from build123d import *

# Parameters (mm, degrees)
SKETCH2_W           = 70
SKETCH2_H           = 50
BOSS_EXTRUDE1_DEPTH = 10
SKETCH3_R           = 4
CUT_EXTRUDE1_DEPTH  = 11
SKETCH4_R           = 2
CUT_EXTRUDE2_DEPTH  = 10
SKETCH5_R           = 8.5
CUT_EXTRUDE3_DEPTH  = 11.0000001


with BuildPart() as part:
    # Sketch2 → Boss-Extrude1 (new body)
    with BuildSketch(Plane(origin=(0, 0, 0), x_dir=(1, 0, 0), z_dir=(0, 1, 0))):
        Rectangle(SKETCH2_W, SKETCH2_H)
    extrude(amount=BOSS_EXTRUDE1_DEPTH)

    # Sketch3 → Cut-Extrude1 (cut, through all)
    with BuildSketch(Plane.XZ):
        with Locations((-25, 15)):
            Circle(SKETCH3_R)
        with Locations((25, 15)):
            Circle(SKETCH3_R)
    extrude(amount=-CUT_EXTRUDE1_DEPTH, mode=Mode.SUBTRACT)

    # Sketch4 → Cut-Extrude2 (cut)
    with BuildSketch(Plane.XY.offset(25)):
        with Locations((25, 5)):
            Circle(SKETCH4_R)
        with Locations((-25, 5)):
            Circle(SKETCH4_R)
    extrude(amount=-CUT_EXTRUDE2_DEPTH, mode=Mode.SUBTRACT)

    # Sketch5 → Cut-Extrude3 (cut, through all)
    with BuildSketch(Plane.XZ):
        with Locations((0, 4)):
            Circle(SKETCH5_R)
    extrude(amount=-CUT_EXTRUDE3_DEPTH, mode=Mode.SUBTRACT)


solid = part.part
Could you check a few things on this model? Use its own coordinates, in mm. A direction names the side the tool comes from. Give positions to 0.01 mm unless a question says otherwise; leave off trailing zeros. Order: outer loops, then holes, each group sorted by start corner. A loop starts at its lowest first (then second) coordinate and runs counter-clockwise, first axis right, second up.
Item 1: I'm going to push flat-ended pins straight in: pin 1 (5 mm diameter, centred on x = -25.5, z = 15.5, fed in from -Y); pin 2 (3 mm diameter, centred on x = 25, y = 5, fed in from +Z). Where does each tip first touch, or does it pass through?
Item 2: If we section it at D-D, the plane y = 1: Write out the boundary of the cut face in (x, z), plus the area to 3 significant figures.
Item 3: I need wall thicknesses on line 1 (X direction, y = 5, z = 20.25); line 2 (Y direction, x = -25, z = 23.25); line 3 (X direction, y = 3.75, z = 11.5). Which ranges of each line are inside material? Lowest first, please.
Item 4: If we mould it in two halves opening along Z, with no side actions, what happens to faces 3 (the face through (4.57, 4.93, 11.167)), 4 (the face through (0, 10, -6)), 5 (the face through (0, 5, 25))? For each: pulls with the +Z half, pulls with the -Z half, needs draft (parallel to the pull), parting line crosses it, or undercut.
Item 5: If we section it at B-B, the plane x = 0: Write out the boundary of the cut face in (y, z), plus the area to 3 significant figures.
Item 6: For faces 1 (the face through (-25, 7, 22)), 2 (the face through (35, 5, 0)), which set-ups out of +Z, -Z, +X, -X, +Y, -Y let a thin tool reach every point of the face, with its end or its side?
Item 7: If we section it at A-A, the plane z = 8: Write out the boundary of the cut face in (x, y), plus the area to 3 significant figures.
Item 8: If we section it at C-C, the plane x = 25: Write out the boundary of the cut face in (y, z).
Values:
1. pin 1: passes through
1. pin 2: stops at z = 11.29
2. outline: (-35, -25) - (35, -25) - (35, 25) - (-35, 25) - close; hole circle Ø8 at (-25, 15); hole circle Ø17 at (0, 4); hole circle Ø8 at (25, 15)
2. area: 3,170 mm2
3. line 1: x = -35 to -27, -23 to 23, 27 to 35
3. line 2: y = 0 to 3, 7 to 10
3. line 3: x = -35 to -26.94, -23.06 to -4, 4 to 23.06, 26.94 to 35
4. face 3: undercut
4. face 4: needs draft
4. face 5: pulls with the +Z half
5. outline: (0, -25) - (10, -25) - (10, -4.5) - (0, -4.5) - close; (0, 12.5) - (10, 12.5) - (10, 25) - (0, 25) - close
5. area: 330 mm2
6. face 1: +Z
6. face 2: +Z, -Z, +X, +Y, -Y
7. outline: (-35, 0) - (-7.5, 0) - (-7.5, 10) - (-35, 10) - close; (7.5, 0) - (35, 0) - (35, 10) - (7.5, 10) - close
7. area: 550 mm2
8. outline: (0, -25) - (10, -25) - (10, 11) - (0, 11) - close; (0, 19) - (3, 19) - (3, 25) - (0, 25) - close; (7, 19) - (10, 19) - (10, 25) - (7, 25) - close
